Input: part model. Units: mm. Frame: model coordinates. Face numbers are marked on the shaded views. Round coordinates to 2 decimals unless told otherwise and drop trailing zeros. Order: outer loops, then holes, each group sorted by start corner. A loop starts at its lowest first (then second) coordinate and runs counter-clockwise, first axis right, second up. Notation, with made-up numbers: (78, 24) - (101, 24) arc R28 ccw to (101, 59) - close; hole circle Ø1 at (35.5, -1). An arc over 180 degrees is marked (long way). One line per item, written item: value. Start each with the question number.
from build123d import *

# Parameters (mm, degrees)
F1_DEPTH = 100
F2_R     = 7
F3_DEPTH = 12.001


with BuildPart() as f1:
    # F0 (on Front) → F1 (new body)
    with BuildSketch(Plane.XZ):
        Polygon((0, 12), (0, 0), (145, 0), (133, 12), align=None)
    extrude(amount=F1_DEPTH)

    # F2 (on Top) → F3 (cut, through all)
    with BuildSketch(Plane.XY):
        with Locations((50, -50)):
            Circle(F2_R)
    extrude(amount=F3_DEPTH, mode=Mode.SUBTRACT)


solid = f1.part
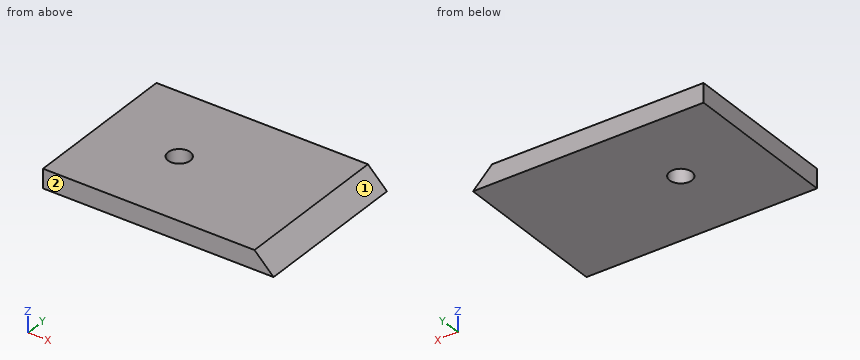
Item 1: Line query: L1, parallel to Y at x = 50, z = 7.5; L2, parallel to X at y = -50, z = 9.5; L3, parallel to X at y = -50, z = 2.5. Output: solid intervals per line, ascending.
Item 2: Section query B-B on y = -50. Return loops of the section in (x, z).
Item 3: Pull-direction query (X, two-part tool) for the marked faces 1 and 2; classes: released by +X, released by -X, zero draft, split by the parting line, or undercut.
Item 4: Section query A-A on x = 50. Return loops of the section in (y, z).
Item 5: First-contact query: pin 1 Ø6 at (y, z) = (-84, 4) entering from +X; pin 2 Ø11 at (x, y) = (50, -50) entering from -Z. Flat tips, straight axial feed; report the tip coordinate or a pass-through.
Item 6: Section query C-C on z = 3.5. Return loops of the section in (x, y).
Item 7: Section query D-D on y = -19.5. Return loops of the section in (x, z), and give its area (3 significant figures).
Geometry results:
1. L1: y = -100 to -57, -43 to 0
1. L2: x = 0 to 43, 57 to 135.5
1. L3: x = 0 to 43, 57 to 142.5
2. outline: (0, 0) - (43, 0) - (43, 12) - (0, 12) - close; (57, 0) - (145, 0) - (133, 12) - (57, 12) - close
3. face 1: released by +X
3. face 2: zero draft
4. outline: (-100, 0) - (-57, 0) - (-57, 12) - (-100, 12) - close; (-43, 0) - (0, 0) - (0, 12) - (-43, 12) - close
5. pin 1: stops at x = 144
5. pin 2: passes through
6. outline: (0, -100) - (141.5, -100) - (141.5, 0) - (0, 0) - close; hole circle Ø14 at (50, -50)
7. outline: (0, 0) - (145, 0) - (133, 12) - (0, 12) - close
7. area: 1,670 mm^2
